```python
from build123d import *

# Parameters (mm, degrees)
SKETCH1_W           = 127
SKETCH1_H           = 203.2
BOSS_EXTRUDE1_DEPTH = 6.0452
SKETCH2_W           = 19.05
SKETCH2_H           = 6.35
BOSS_EXTRUDE2_DEPTH = 6.0452
SKETCH3_W           = 8.6868
SKETCH3_H           = 19.05
BOSS_EXTRUDE3_DEPTH = 6.0452


with BuildPart() as part:
    # Sketch1 → Boss-Extrude1 (new body)
    with BuildSketch(Plane.XY):
        Rectangle(SKETCH1_W, SKETCH1_H)
    extrude(amount=BOSS_EXTRUDE1_DEPTH)

    # Sketch2 → Boss-Extrude2 (add)
    with BuildSketch(Plane.XY.offset(6.0452)):
        with Locations((0, 101.6)):
            Rectangle(SKETCH2_W, SKETCH2_H)
        with Locations((-38.1, 101.6)):
            Rectangle(SKETCH2_W, SKETCH2_H)
        with Locations((38.1, 101.6)):
            Rectangle(SKETCH2_W, SKETCH2_H)
        with Locations((38.1, -101.6)):
            Rectangle(SKETCH2_W, SKETCH2_H)
        with Locations((-38.1, -101.6)):
            Rectangle(SKETCH2_W, SKETCH2_H)
        with Locations((0, -101.6)):
            Rectangle(SKETCH2_W, SKETCH2_H)
    extrude(amount=-BOSS_EXTRUDE2_DEPTH)

    # Sketch3 → Boss-Extrude3 (add)
    with BuildSketch(Plane.XY.offset(6.0452)):
        with Locations((63.5, 0)):
            Rectangle(SKETCH3_W, SKETCH3_H)
        with Locations((63.5, 35.052)):
            Rectangle(SKETCH3_W, SKETCH3_H)
        with Locations((63.5, 70.104)):
            Rectangle(SKETCH3_W, SKETCH3_H)
        with Locations((63.5, -70.104)):
            Rectangle(SKETCH3_W, SKETCH3_H)
        with Locations((63.5, -35.052)):
            Rectangle(SKETCH3_W, SKETCH3_H)
        with Locations((-63.5, -35.052)):
            Rectangle(SKETCH3_W, SKETCH3_H)
        with Locations((-63.5, -70.104)):
            Rectangle(SKETCH3_W, SKETCH3_H)
        with Locations((-63.5, 70.104)):
            Rectangle(SKETCH3_W, SKETCH3_H)
        with Locations((-63.5, 35.052)):
            Rectangle(SKETCH3_W, SKETCH3_H)
        with Locations((-63.5, 0)):
            Rectangle(SKETCH3_W, SKETCH3_H)
    extrude(amount=-BOSS_EXTRUDE3_DEPTH)


solid = part.part
```
The model under review builds one solid part; all positions refer to its coordinate system, in mm. A direction names the side the tool comes from. Give positions to 0.01 mm unless a question says otherwise; leave off trailing zeros. Order: outer loops, then holes, each group sorted by start corner. A loop starts at its lowest first (then second) coordinate and runs counter-clockwise, first axis right, second up. Notation, with made-up numbers: (17.5, -29.75) - (49.5, -29.75) arc R18 cw to (49.5, -15.75) - close; hole circle Ø2 at (-26, 71). An arc over 180 degrees is marked (long way). Use CSV: the item, a comma, the result in double quotes. Start each with the question number.
Q1. Clearance check with flat-ended pins moving along their axes: pin 1 Ø1.5 at (x, z) = (22.5, 4.5) entering from +Y; pin 2 Ø2.5 at (y, z) = (103, 4) entering from -X (3 decimals); pin 3 Ø4 at (x, y) = (16, 39.5) entering from -Z; pin 4 Ø1.8 at (x, z) = (-58.5, 4.5) entering from -Y. State where each tip first meets the part, or that it passes through.
Q2. We need section A-A, the plane y = -50.5. Write out the cut boundary in (x, z).
Q3. We need section B-B, the plane x = 13.5. Write out the cut boundary in (y, z).
Q4. Tool access review of faces 1 (the flat face through (63.5, 90, 3)), 2 (the flat face through (66, 44.577, 3)), 3 (the flat face through (-66, -60.579, 3)): name each direction out of +Z, -Z, +X, -X, +Y, -Y from which nothing blocks a thin tool from reaching the whole face with its end or side.
Q5. The part is to be moulded in two halves that separate along X. For faces 4 (the flat face through (19, -101.6, 3)), 5 (the flat face through (-56, -101.6, 3)), 6 (the flat face through (-67.843, 0, 3)), say which applies: +X half, -X half, draft (parallel to the pull), parting line (faces both ways), or undercut.
Q6. To check wall thickness, follow line 1 along X through (y, z) = (94, 5.25); line 2 along Y through (x, z) = (-11, 0.75). State the ranges of each line that lie inside material, in increasing order. Write a range as [from, to].
Outcome:
1,pin 1,"stops at y = 101.6"
1,pin 2,"stops at x = -47.625"
1,pin 3,"stops at z = 0"
1,pin 4,"stops at y = -101.6"
2,outline,"(-63.5, 0) - (63.5, 0) - (63.5, 6.05) - (-63.5, 6.05) - close"
3,outline,"(-101.6, 0) - (101.6, 0) - (101.6, 6.05) - (-101.6, 6.05) - close"
4,face 1,"+Z, -Z, +X, +Y"
4,face 2,"+Z, -Z, +X"
4,face 3,"+Z, -Z, -X"
5,face 4,"undercut"
5,face 5,"draft"
5,face 6,"-X half"
6,line 1,"x = [-63.5, 63.5]"
6,line 2,"y = [-101.6, 101.6]"
